Model file for the job. Use its own axes, mm. A direction names the side the tool comes from. Coordinates: 2 decimals unless noted, no trailing zeros. Order: outer loops, then holes, each group sorted by start corner. A loop starts at its lowest first (then second) coordinate and runs counter-clockwise, first axis right, second up. Notation, with made-up numbers: (-1, 69) -> (36, 69) arc R36 ccw to (36, 103) -> close; hole circle Ø6 at (31.25, 80.5). An arc over 180 degrees is marked (long way). Use CSV: the item, a comma, the result in double quotes. Start each with the question number.
(1) Pin check, flat tips, straight feed: pin 1 Ø2 at (x, y) = (3, 7.5) entering from +Z; pin 2 Ø5.5 at (x, y) = (24.5, -1) entering from -Z; pin 3 Ø1.8 at (x, z) = (25.5, 6.5) entering from -Y; pin 4 Ø12 at (x, y) = (-12, 3) entering from -Z. Stop position of each tip, or through.
(2) Cut at D-D on x = 26. Write the cut outline in (y, z).
(3) Tool access for faces 4 (the flat face through (26, 0, 5.9)), 5 (the flat face through (25, -5.5, 7)), 6 (the cylindrical face through (0.284, 11.449, 0.285)): list every direction of +Z, -Z, +X, -X, +Y, -Y with a clear straight run to the whole face (end or side of a thin tool).
(4) Cut at B-B on y = 0. Write the cut outline in (x, z), plus the area to 3 significant figures.
(5) Pull direction X, two halves, no side cores. Call faces 1 (the flat face through (26, 0, 7.5)), 2 (the cylindrical face through (21.68, 11.15, 10.89)), 3 (the flat face through (0, 0, 21.5)): pulls with the +X half, pulls with the -X half, needs draft (parallel to the pull), parting line crosses it, or undercut.
(6) Cut at A-A on z = 3.75. Write the cut outline in (x, y), plus the area to 3 significant figures.
(7) Cut at C-C on z = 6.5. Write the cut outline in (x, y).
(8) Probe L1, parallel to X at y = -0.5, z = 16.5; L2, parallel to Z at x = 21, y = 8.5; L3, parallel to Y at x = 21, z = 3.25. List the from-to ranges inside material, lowest first.
Autodesk Inventor part; units mm, degrees
ref_plane "YZ Plane" through (0, 0, 0) normal (1, 0, 0) x (0, 1, 0)
ref_plane "XZ Plane" through (0, 0, 0) normal (0, 1, 0) x (-1, 0, 0)
ref_plane "XY Plane" through (0, 0, 0) normal (0, 0, 1) x (1, 0, 0)
sketch "Sketch2" plane through (0, 0, 0) normal (0, 0, 1) x (1, 0, 0)
  line L0 (22.25, -11.75) -> (-22.25, -11.75)
  line L1 (-22.25, -11.75) -> (-22.25, 11.75)
  line L2 (-22.25, 11.75) -> (22.25, 11.75)
  line L3 (22.25, 11.75) -> (22.25, -11.75)
  line L4 (22.25, -11.75) -> (-22.25, 11.75) construction
  line L5 (-22.25, -11.75) -> (22.25, 11.75) construction
  point P0 (0, 0)
  dimension "d0" = 44.5
  dimension "d1" = 23.5
extrude "Extrusion1" add sketch "Sketch2" along normal blind 21.5
sketch "Sketch3" plane through (22.25, -11.75, 0) normal (1, 0, 0) x (0, 0, -1)
  line L0 (-7.5, 17.25) -> (-5.9, 17.25)
  line L1 (-5.9, 17.25) -> (-5.9, 6.25)
  line L2 (-5.9, 6.25) -> (-7.5, 6.25)
  line L3 (-7.5, 6.25) -> (-7.5, 17.25)
  line L4 (-21.5, 0) -> (-21.5, 23.5) construction
  line L5 (0, 23.5) -> (-21.5, 23.5) construction
  point P0 (0, 11.75)
  dimension "d4" = 11
  dimension "d5" = 1.6
  dimension "d6" = 14
  dimension "d7" = 6.25
  dimension "d8" = 23.5
extrude "Extrusion2" add sketch "Sketch3" along normal blind 7
sketch "Sketch4" plane through (0, 0, 21.5) normal (0, 0, 1) x (1, 0, 0)
  line L0 (22.25, 11.75) -> (-22.25, 11.75) construction
  line L1 (-22.25, 11.75) -> (-22.25, -11.75) construction
  line L2 (-22.25, -11.75) -> (22.25, -11.75) construction
  line L3 (22.25, -11.75) -> (22.25, 11.75) construction
  circle A0 centre (-10, 0) radius 9
  circle A1 centre (10, 0) radius 9
  line L4 (0, 16.45) -> (0, -16.45) construction
  line L5 (-33.55, 0) -> (45.55, 0) construction
  point P0 (0, 0)
  dimension "d11" = 18
  dimension "d12" = 10
  dimension "d13" = 18
  dimension "d14" = 10
extrude "Extrusion3" add sketch "Sketch4" along normal blind 0.1
fillet "Fillet1" radius 2 4 edges at (-22.25, 11.75, 10.75) (22.25, 11.75, 10.75) (22.25, -11.75, 10.75) (-22.25, -11.75, 10.75)
fillet "Fillet2" radius 1 18 edges at (-21.6642, 11.1642, 21.5) (-22.25, 0, 21.5) (-21.6642, -11.1642, 21.5) (0, -11.75, 21.5) (21.6642, -11.1642, 21.5) (22.25, 0, 21.5) (21.6642, 11.1642, 21.5) (0, 11.75, 21.5) (-21.6642, 11.1642, 0) (-22.25, 0, 0) (-21.6642, -11.1642, 0) (0, -11.75, 0) (21.6642, -11.1642, 0) (22.25, 0, 0) (21.6642, 11.1642, 0) (0, 11.75, 0) (29.25, 5.5, 6.7) (29.25, -5.5, 6.7)
sketch "Sketch5" plane through (-20.25, 11.75, 1) normal (0, 1, 0) x (1, 0, 0)
  point P0 (20.25, 1)
equation "\"d7\" = -0.5 * d4 + 0.5 * d8"
properties part number "P041_Lidar"
Outcome:
1,pin 1,"z = 21.5"
1,pin 2,"z = 0.13"
1,pin 3,"y = -5.5"
1,pin 4,"z = 0"
2,outline,"(-5.5, 5.9) -> (5.5, 5.9) -> (5.5, 7.5) -> (-5.5, 7.5) -> close"
3,face 4,"-Z, +X, +Y, -Y"
3,face 5,"+Z, -Z, +X, -Y"
3,face 6,"-Z, +X, -X, +Y"
4,outline,"(-22.25, 1) arc R1 ccw to (-21.25, 0) -> (21.25, 0) arc R1 ccw to (22.25, 1) -> (22.25, 5.9) -> (29.25, 5.9) -> (29.25, 7.5) -> (22.25, 7.5) -> (22.25, 20.5) arc R1 ccw to (21.25, 21.5) -> (19, 21.5) -> (19, 21.6) -> (1, 21.6) -> (1, 21.5) -> (-1, 21.5) -> (-1, 21.6) -> (-19, 21.6) -> (-19, 21.5) -> (-21.25, 21.5) arc R1 ccw to (-22.25, 20.5) -> close"
4,area,"971 mm2"
5,face 1,"needs draft"
5,face 2,"pulls with the +X half"
5,face 3,"undercut"
6,outline,"(-22.25, -9.75) arc R2 ccw to (-20.25, -11.75) -> (20.25, -11.75) arc R2 ccw to (22.25, -9.75) -> (22.25, 9.75) arc R2 ccw to (20.25, 11.75) -> (-20.25, 11.75) arc R2 ccw to (-22.25, 9.75) -> close"
6,area,"1,040 mm2"
7,outline,"(-22.25, -9.75) arc R2 ccw to (-20.25, -11.75) -> (20.25, -11.75) arc R2 ccw to (22.25, -9.75) -> (22.25, -5.5) -> (28.25, -5.5) arc R1 ccw to (29.25, -4.5) -> (29.25, 4.5) arc R1 ccw to (28.25, 5.5) -> (22.25, 5.5) -> (22.25, 9.75) arc R2 ccw to (20.25, 11.75) -> (-20.25, 11.75) arc R2 ccw to (-22.25, 9.75) -> close"
8,L1,"-22.25 to 22.25"
8,L2,"0 to 21.5"
8,L3,"-11.6 to 11.6"
